Can you work these out from the model? Positions are in its coordinate system, mm. A direction names the side the tool comes from. Coordinates: 2 decimals unless noted, no trailing zeros. Loops run counter-clockwise (first coordinate to the right, second up) from the corner with the lowest first, then second, coordinate; pieces in that order, holes last. Notation, with made-up numbers: (28.5, -36) -> (39.5, -36) arc R12 cw to (39.5, -13) -> close; hole circle Ø2 at (82.5, -20.5). An arc over 180 degrees is marked (long way). Put each result on its own line as item: value. Start each with the question number.
Item 1: If we section it at D-D on z = 40: Please give me the cut outline in (x, y) (3 decimals).
Item 2: Please list where these lines run through material, in increasing order: L1, parallel to Y at x = 14.5, z = 57 (3 decimals); L2, parallel to Y at x = -49.5, z = -45 (3 decimals); L3, parallel to X at y = 3.5, z = -23.5. Write a range as from..to.
Item 3: If we section it at B-B on z = -9: Please give me the cut outline in (x, y) (3 decimals).
Item 4: For faces 4 (the cylindrical face through (-20.653, 0.089, -59.052)), 5 (the flat face through (-2, 15.875, 12)), 6 (the cylindrical face through (-112.794, -0.222, -4.15)), 7 (the flat face through (77, 0, -56.626)), which set-ups out of +Z, -Z, +X, -X, +Y, -Y let a thin tool reach every point of the face, with its end or its side?
Item 5: We'd pull the mould along X, two halves only. Please class faces 1 (the cylindrical face through (116.074, -0.877, 57.852)), 2 (the cylindrical face through (42.844, -0.19, -4.759)), 3 (the flat face through (-2, -15.875, 12)): pulls with the +X half, pulls with the -X half, needs draft (parallel to the pull), parting line crosses it, or undercut.
Item 6: Will these pins go through, and if not, where does the flat tip stop? P1, Ø4, axis at x = -37, z = 44.5, coming from the -Y side (3 decimals); P2, Ø8, axis at x = -72, y = 13, coming from the +Z side; P3, Ø5, axis at y = -4.5, z = 27, coming from the +X side.
Item 7: If we section it at C-C on y = 10: Please give me the cut outline in (x, z), plus the area to 3 significant figures.
Item 8: If we section it at A-A on x = 55: Please give me the cut outline in (y, z) (3 decimals).
```python
from build123d import *

# Parameters (mm, degrees)
F0_R     = 38.1
F1_DEPTH = 15.875
F3_DEPTH = 152.4
F4_R     = 12.7
F5_DEPTH = 25.4


# Not quite as in the source:
# - a feature names something its author has since deleted; it is built from what else it names


with BuildPart() as f1:
    # F0 (on Front) → F1 (new body, symmetric)
    with BuildSketch(Plane.XZ):
        with BuildLine():
            Line((70.8614879427, 70.3741200164), (-36.6122665732, 70.3741200164))
            ThreePointArc((-36.6122665732, 70.3741200164), (-112.8122614121, -5.8258799836), (-36.6122665732, -82.0258799836))
            Line((-36.6122665732, -82.0258799836), (70.8614879427, -82.0258799836))
            Line((70.8614879427, -82.0258799836), (70.8614879427, -56.6258799836))
            Line((70.8614879427, -56.6258799836), (52.2877385879, -56.6258799836))
            Line((52.2877385879, -56.6258799836), (52.2877385879, 44.9741200164))
            Line((52.2877385879, 44.9741200164), (70.8614879427, 44.9741200164))
            Line((70.8614879427, 44.9741200164), (70.8614879427, 70.3741200164))
        make_face()
        with Locations((-36.6122614121, -5.8258799836)):
            Circle(F0_R, mode=Mode.SUBTRACT)
    extrude(amount=F1_DEPTH, both=True)

    # F2 (on face) → F3 (cut)
    with BuildSketch(Plane.XY.offset(70.3741200164)):
        with BuildLine():
            Line((36.4952879427, 6.2992834322), (-14.3047120573, 6.2992834322))
            ThreePointArc((-14.3047120573, 6.2992834322), (-20.6547120573, -0.0507165678), (-14.3047120573, -6.4007165678))
            Line((-14.3047120573, -6.4007165678), (36.4952879427, -6.4007165678))
            ThreePointArc((36.4952879427, -6.4007165678), (42.8452879427, -0.0507165678), (36.4952879427, 6.2992834322))
        make_face()
    extrude(amount=-F3_DEPTH, mode=Mode.SUBTRACT)

    # F4 (on face) → F5 (join)
    with BuildSketch(Plane.XY.offset(70.3741200164)):
        with BuildLine():
            Line((70.8614879427, 15.875), (70.8614879427, -15.875))
            ThreePointArc((70.8614879427, -15.875), (116.0893565876, 0), (70.8614879427, 15.875))
        make_face()
        with Locations((90.6893565876, 0)):
            Circle(F4_R, mode=Mode.SUBTRACT)
    extrude(amount=-F5_DEPTH)

    # F7: F1 across plane


with BuildPart() as f1_1:
    add(f1.part)
    add(f1.part.mirror(Plane(origin=(52.2877385879, -15.875, -5.8258799836), x_dir=(1, 0, 0), z_dir=(0, 0, -1))))


solid = f1_1.part
```
Solutions:
1. outline: (-97.493, -15.875) -> (52.288, -15.875) -> (52.288, 15.875) -> (-97.493, 15.875) -> close; hole (-14.305, -6.401) -> (36.495, -6.401) arc R6.35 ccw to (36.495, 6.299) -> (-14.305, 6.299) arc R6.35 ccw to start
2. L1: -15.875..-6.401, 6.299..15.875
2. L2: -15.875..15.875
2. L3: -110.73..-70.36, 41.76..52.29
3. outline: (-112.746, -15.875) -> (-74.58, -15.875) -> (-74.58, 15.875) -> (-112.746, 15.875) -> close; (1.355, -15.875) -> (52.288, -15.875) -> (52.288, 15.875) -> (1.355, 15.875) -> (1.355, 6.299) -> (36.495, 6.299) arc R6.35 cw to (36.495, -6.401) -> (1.355, -6.401) -> close
4. face 4: +Z, -Z
4. face 5: +Z, -Z, -X, +Y
4. face 6: -X, +Y, -Y
4. face 7: +X, +Y, -Y
5. face 1: parting line crosses it
5. face 2: undercut
5. face 3: needs draft
6. P1: y = -15.875
6. P2: z = 63.61
6. P3: x = 52.29
7. outline: (-36.61, -82.03) -> (82.86, -82.03) -> (82.86, -56.63) -> (52.29, -56.63) -> (52.29, 44.97) -> (82.86, 44.97) -> (82.86, 70.37) -> (-36.61, 70.37) arc R76.2 ccw to start; (98.52, -82.03) -> (114.04, -82.03) -> (114.04, -56.63) -> (98.52, -56.63) -> close; (98.52, 44.97) -> (114.04, 44.97) -> (114.04, 70.37) -> (98.52, 70.37) -> close; hole circle Ø76.2 at (-36.61, -5.83)
7. area: 20,500 mm^2
8. outline: (-15.875, -82.026) -> (15.875, -82.026) -> (15.875, -56.626) -> (-15.875, -56.626) -> close; (-15.875, 44.974) -> (15.875, 44.974) -> (15.875, 70.374) -> (-15.875, 70.374) -> close
